Read the model definition and answer for the solid it produces. Units are mm, in the model's axes. Face numbers are marked on the shaded views. Give positions to 0.01 mm unless a question says otherwise; leave off trailing zeros. Write each loop counter-clockwise with the first axis right and the second up, starting at its lowest first coordinate (ties: lowest second). Pieces come first, ordered by that corner, then holes. Notation, with made-up numbers: (41, 69.25) -> (54, 69.25) arc R20 cw to (54, 100.25) -> close; hole circle Ø7 at (17.5, 33.25). An arc over 180 degrees is marked (long way). Write item = value, one per line.
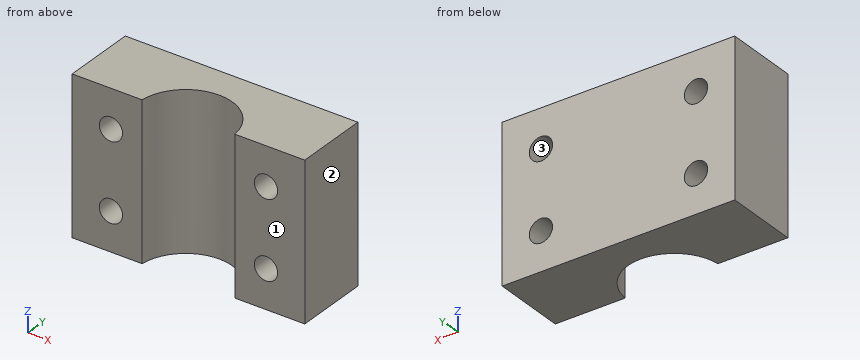
from build123d import *

# Parameters (mm, degrees)
BOSS_EXTRU_1_DEPTH      = 20
ESQUISSE3_R             = 1.5
ENL_V_MAT_EXTRU_1_DEPTH = 10


with BuildPart() as part:
    # Esquisse2 → Boss.-Extru.1 (new body)
    with BuildSketch(Plane.XY):
        with BuildLine():
            Line((-15, 0.5), (-15, 10))
            Line((-15, 10), (15, 10))
            Line((15, 10), (15, 0.5))
            Line((15, 0.5), (5.979130372, 0.5))
            ThreePointArc((5.979130372, 0.5), (0, 6), (-5.979130372, 0.5))
            Line((-5.979130372, 0.5), (-15, 0.5))
        make_face()
    extrude(amount=BOSS_EXTRU_1_DEPTH)

    # Esquisse3 → Enlèv. mat.-Extru.1 (cut)
    with BuildSketch(Plane(origin=(0, 10, 0), x_dir=(1, 0, 0), z_dir=(0, 1, 0))):
        with Locations((-10, -5)):
            Circle(ESQUISSE3_R)
        with Locations((10, -5)):
            Circle(ESQUISSE3_R)
        with Locations((-10, -15)):
            Circle(ESQUISSE3_R)
        with Locations((10, -15)):
            Circle(ESQUISSE3_R)
    extrude(amount=-ENL_V_MAT_EXTRU_1_DEPTH, mode=Mode.SUBTRACT)


solid = part.part
(1) Consider L1, parallel to Z at x = -10, y = 2.5; L2, parallel to X at y = 8, z = 5; L3, parallel to X at y = 3.25, z = 5. Determine where each line is inside the solid, lowest interval first.
Checks:
L1 = 0 to 3.5, 6.5 to 13.5, 16.5 to 20
L2 = -15 to -11.5, -8.5 to 8.5, 11.5 to 15
L3 = -15 to -11.5, -8.5 to -5.04, 5.04 to 8.5, 11.5 to 15
(2) The part is cut by section B-B on y = 3. Determine the outline of the cut face in (x, z).
Checks:
outline = (-15, 0) -> (-5.2, 0) -> (-5.2, 20) -> (-15, 20) -> close; (5.2, 0) -> (15, 0) -> (15, 20) -> (5.2, 20) -> close; hole circle Ø3 at (-10, 5); hole circle Ø3 at (-10, 15); hole circle Ø3 at (10, 5); hole circle Ø3 at (10, 15)
(3) For a pull along X with two mould halves and no side action, classify the marked faces 1, 2 and 3 as released by +X, released by -X, zero draft, split by the parting line, or undercut.
Checks:
face_1 = zero draft
face_2 = released by +X
face_3 = undercut
(4) The part is cut by section C-C on x = -10. Determine the outline of the cut face in (y, z), plus the area to 3 significant figures.
Checks:
outline = (0.5, 0) -> (10, 0) -> (10, 3.5) -> (0.5, 3.5) -> close; (0.5, 6.5) -> (10, 6.5) -> (10, 13.5) -> (0.5, 13.5) -> close; (0.5, 16.5) -> (10, 16.5) -> (10, 20) -> (0.5, 20) -> close
area = 133 mm²
(5) The part is cut by section A-A on z = 5. Determine the outline of the cut face in (x, y).
Checks:
outline = (-15, 0.5) -> (-11.5, 0.5) -> (-11.5, 10) -> (-15, 10) -> close; (-8.5, 0.5) -> (-5.98, 0.5) arc R6 cw to (5.98, 0.5) -> (8.5, 0.5) -> (8.5, 10) -> (-8.5, 10) -> close; (11.5, 0.5) -> (15, 0.5) -> (15, 10) -> (11.5, 10) -> close
(6) Given P1, Ø5, axis at x = -5, y = 2, coming from the -Z side; P2, Ø2.5, axis at x = 10, z = 5, coming from the +Y side, each flat-ended and moving along its own axis, determine where each tip first touches the part or whether it passes through.
Checks:
P1 = 0
P2 = through
(7) The part is cut by section D-D on y = 7.5. Determine the outline of the cut face in (x, z).
Checks:
outline = (-15, 0) -> (15, 0) -> (15, 20) -> (-15, 20) -> close; hole circle Ø3 at (-10, 5); hole circle Ø3 at (-10, 15); hole circle Ø3 at (10, 5); hole circle Ø3 at (10, 15)
